from build123d import *

# Parameters (mm, degrees)
SKETCH1_R           = 5
SKETCH1_R_2         = 3
BOSS_EXTRUDE1_DEPTH = 6
SKETCH5_R           = 5
BOSS_EXTRUDE5_DEPTH = 2
SKETCH7_R           = 3.75
BOSS_EXTRUDE6_DEPTH = 2


with BuildPart() as part:
    # Sketch1 → Boss-Extrude1 (new body)
    # profile 1 of 3: a face of its own
    with BuildSketch(Plane(origin=(0, 0, 0), x_dir=(1, 0, 0), z_dir=(0, 1, 0))):
        with Locations(Location((0, 0, 0), (0, 0, 270))):
            Circle(SKETCH1_R)
        Circle(SKETCH1_R_2, mode=Mode.SUBTRACT)
    # profile 2 of 3: a face of its own
    with BuildSketch(Plane(origin=(0, 0, 0), x_dir=(1, 0, 0), z_dir=(0, 1, 0))):
        with BuildLine():
            Line((2.436698586, -1.75), (-2.436698586, -1.75))
            ThreePointArc((-2.436698586, -1.75), (0, -3), (2.436698586, -1.75))
        make_face()
    # profile 3 of 3: a face of its own
    with BuildSketch(Plane(origin=(0, 0, 0), x_dir=(1, 0, 0), z_dir=(0, 1, 0))):
        with BuildLine():
            ThreePointArc((2.436698586, 1.75), (0, 3), (-2.436698586, 1.75))
            Line((-2.436698586, 1.75), (2.436698586, 1.75))
        make_face()
    extrude(amount=BOSS_EXTRUDE1_DEPTH)

    # Sketch5 → Boss-Extrude5 (add)
    with BuildSketch(Plane(origin=(0, 6, 0), x_dir=(1, 0, 0), z_dir=(0, 1, 0))):
        with Locations(Location((0, 0, 0), (0, 0, 270))):
            Circle(SKETCH5_R)
    extrude(amount=BOSS_EXTRUDE5_DEPTH)

    # Sketch7 → Boss-Extrude6 (add)
    with BuildSketch(Plane(origin=(0, 8, 0), x_dir=(1, 0, 0), z_dir=(0, 1, 0))):
        with Locations(Location((0, 0, 0), (0, 0, 270))):
            Circle(SKETCH7_R)
    extrude(amount=BOSS_EXTRUDE6_DEPTH)


solid = part.part
Input: part model. Units: mm. Frame: model coordinates. A direction names the side the tool comes from. Coordinates: 2 decimals unless noted, no trailing zeros. Write each loop counter-clockwise with the first axis right and the second up, starting at its lowest first coordinate (ties: lowest second). Pieces come first, ordered by that corner, then holes. Notation, with made-up numbers: M 4.25,58 L 22.25,58 A16 cw 22.25,63 Z; hole C -6,5 d8. An arc over 180 degrees is marked long. Answer as a JSON object with one key per item and string values. Group by question number.
(1) Mould query, pull axis Z, two halves, no side actions, for faces 1 (the face through (3, 3, 0)), 2 (the face through (0.165, 8.986, -3.746)), 3 (the face through (0, 3, 1.75)), 4 (the face through (0, 10, 0)). Classes: pulls with the +Z half, pulls with the -Z half, needs draft (parallel to the pull), parting line crosses it, or undercut.
(2) Section A-A on y = 4.25. Output: boundary loops of the cut face in (x, z).
(3) Section D-D on x = 4. Output: boundary loops of the cut face in (y, z).
(4) Section B-B on x = 0. Output: boundary loops of the cut face in (y, z), plus the area to 3 significant figures.
(5) Ray query, line 1 along Z through (x, y) = (4, 5); line 2 along Z through (x, y) = (-2.75, 1.25). Return the intervals inside material, ascending. Write a range as [from, to].
(6) Set-up query: faces 5 (the face through (4, 8, 1)), 6 (the face through (-4.88, 3.94, -1.08)), 7 (the face through (0, 3, -1.75)). Return all of +Z, -Z, +X, -X, +Y, -Y with unobstructed straight access to the full face (end or side cutting, diameter ignored); none if empty.
(7) Section C-C on z = 0. Output: boundary loops of the cut face in (x, y), plus the area to 3 significant figures.
(8) Contact query for flat-ended pins moving along their axis: P1, Ø1.5, axis at x = -1, y = 1.5, coming from the +Z side; P2, Ø1.5, axis at x = 1.5, y = 7.5, coming from the -Z side. Output: stop coordinate, or through.
Result set:
{
 "1": {"face 1": "undercut", "face 2": "parting line crosses it", "face 3": "undercut", "face 4": "needs draft"},
 "2": {"outline": "C 0,0 d10; hole M -2.44,-1.75 L 2.44,-1.75 A3 ccw 2.44,1.75 L -2.44,1.75 A3 ccw Z"},
 "3": {"outline": "M 0,-3 L 8,-3 L 8,3 L 0,3 Z"},
 "4": {"outline": "M 0,-5 L 8,-5 L 8,-3.75 L 10,-3.75 L 10,3.75 L 8,3.75 L 8,5 L 0,5 L 0,1.75 L 6,1.75 L 6,-1.75 L 0,-1.75 Z", "area": "74.0 mm2"},
 "5": {"line 1": "z = [-3, 3]", "line 2": "z = [-4.18, -1.2], [1.2, 4.18]"},
 "6": {"face 5": "+Y", "face 6": "+Y, -Y", "face 7": "-Y"},
 "7": {"outline": "M -5,0 L -3,0 L -3,6 L 3,6 L 3,0 L 5,0 L 5,8 L 3.75,8 L 3.75,10 L -3.75,10 L -3.75,8 L -5,8 Z", "area": "59.0 mm2"},
 "8": {"P1": "stops at z = 4.99", "P2": "stops at z = -4.94"}
}
